Source: CAD feature listing. Evaluate the final solid. Frame: model axes, mm. Face numbers are marked on the shaded views. A direction names the side the tool comes from. Round coordinates to 2 decimals unless told otherwise and drop trailing zeros. Order: outer loops, then holes, each group sorted by start corner. A loop starts at its lowest first (then second) coordinate and runs counter-clockwise, first axis right, second up. Notation, with made-up numbers: (-2.75, 43) -> (40.25, 43) arc R10 ccw to (40.25, 49) -> close; hole circle Ø1 at (19, 37.5). An arc over 180 degrees is marked (long way). Answer as CSV lines item,"result". Start each with the question number.
(1) Set-up query: the marked faces 1 and 2. Return all of +Z, -Z, +X, -X, +Y, -Y with unobstructed straight access to the full face (end or side cutting, diameter ignored); none if empty.
(2) Section query D-D (z = 17.5). Output: boundary loops of the cut face in (x, y).
(3) Contact query for flat-ended pins moving along their axis: P1, Ø12, axis at y = -43.5, z = 64, coming from the -X side; P2, Ø4, axis at x = -90, y = -11, coming from the +Z side; P3, Ø10, axis at x = -128.5, y = -52.5, coming from the +Z side. Output: stop coordinate, or through.
(4) Section query A-A (x = -32). Output: boundary loops of the cut face in (y, z), plus the area to 3 significant figures.
(5) Pull-direction query (Z, two-part tool) for the marked faces 3, 4 and 5; classes: +Z half, -Z half, draft (parallel to the pull), parting line (faces both ways), or undercut.
(6) Section query C-C (y = -56.5). Output: boundary loops of the cut face in (x, z).
(7) Section query B-B (z = 63). Output: boundary loops of the cut face in (x, y).
(8) Line query: line 1 along X through (y, z) = (-7, 64); line 2 along X through (y, z) = (-75.5, 13); line 3 along Z through (x, y) = (-66.5, -90.5). Output: solid intervals per line, ascending. Write a range as from..to.
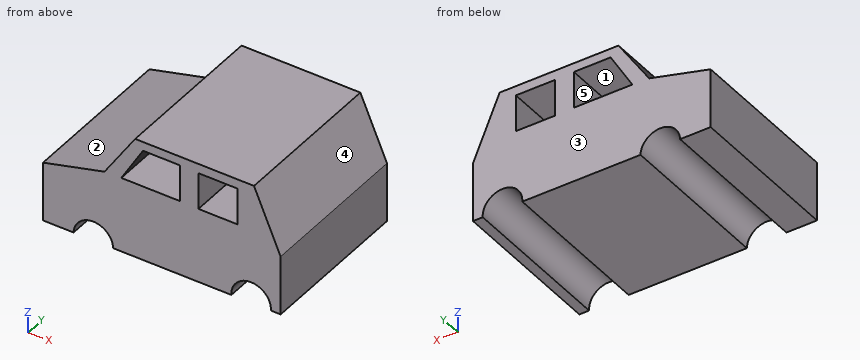
```python
from build123d import *

# Parameters (mm, degrees)
F1_DEPTH = 101.6
F3_DEPTH = 115.062
F4_W     = 25.222163
F4_H     = 23.562811
F5_DEPTH = 157.988
F6_R     = 12.7
F7_DEPTH = 195.834
F8_R     = 12.7
F9_DEPTH = 145.542


with BuildPart() as f1:
    # F0 (on Front) → F1 (new body)
    with BuildSketch(Plane.XZ):
        Polygon((-105.85011, 56.459235), (-145.276219, 46.419184), (-145.276219, 8.319184), (7.123781, 8.319184), (7.123781, 46.419184), (-9.965162, 86.073698), (-86.165162, 86.073698), align=None)
    extrude(amount=F1_DEPTH)

    # F2 (on Front) → F3 (cut)
    with BuildSketch(Plane.XZ):
        Polygon((-81.123598, 80.316171), (-95.062166, 56.75336), (-57.560787, 56.75336), (-57.560787, 80.316171), align=None)
    extrude(amount=F3_DEPTH, mode=Mode.SUBTRACT)

    # F4 (on Front) → F5 (cut)
    with BuildSketch(Plane.XZ):
        with Locations((-33.002364, 68.202894)):
            Rectangle(F4_W, F4_H)
    extrude(amount=F5_DEPTH, mode=Mode.SUBTRACT)

    # F6 (on Front) → F7 (cut)
    with BuildSketch(Plane.XZ):
        with Locations((-112.983182, 7.968382)):
            Circle(F6_R)
    extrude(amount=F7_DEPTH, mode=Mode.SUBTRACT)

    # F8 (on Front) → F9 (cut)
    with BuildSketch(Plane.XZ):
        with Locations((-11.795502, 9.144407)):
            Circle(F8_R)
    extrude(amount=F9_DEPTH, mode=Mode.SUBTRACT)


solid = f1.part
```
Answer block:
1,face 1,"+Y, -Y"
1,face 2,"+Z, -X, +Y, -Y"
2,outline,"(-145.28, -101.6) -> (-121.38, -101.6) -> (-121.38, 0) -> (-145.28, 0) -> close; (-104.59, -101.6) -> (-21.36, -101.6) -> (-21.36, 0) -> (-104.59, 0) -> close; (-2.23, -101.6) -> (7.12, -101.6) -> (7.12, 0) -> (-2.23, 0) -> close"
3,P1,"x = -104.83"
3,P2,"z = 83.31"
3,P3,"z = 51.96"
4,outline,"(-101.6, 8.32) -> (0, 8.32) -> (0, 56.42) -> (-101.6, 56.42) -> close; (-101.6, 79.98) -> (0, 79.98) -> (0, 86.07) -> (-101.6, 86.07) -> close"
4,area,"5,510 mm2"
5,face 3,"draft"
5,face 4,"+Z half"
5,face 5,"undercut"
6,outline,"(-145.28, 8.32) -> (-125.68, 8.32) arc R12.7 cw to (-100.29, 8.32) -> (-24.47, 8.32) arc R12.7 cw (long way) to (0.88, 8.32) -> (7.12, 8.32) -> (7.12, 46.42) -> (-9.97, 86.07) -> (-86.17, 86.07) -> (-105.85, 56.46) -> (-145.28, 46.42) -> close; hole (-95.06, 56.75) -> (-57.56, 56.75) -> (-57.56, 80.32) -> (-81.12, 80.32) -> close; hole (-45.61, 56.42) -> (-20.39, 56.42) -> (-20.39, 79.98) -> (-45.61, 79.98) -> close"
7,outline,"(-101.5, -101.6) -> (-91.37, -101.6) -> (-91.37, 0) -> (-101.5, 0) -> close; (-57.56, -101.6) -> (-45.61, -101.6) -> (-45.61, 0) -> (-57.56, 0) -> close; (-20.39, -101.6) -> (-0.02, -101.6) -> (-0.02, 0) -> (-20.39, 0) -> close"
8,line 1,"-100.84..-90.78, -57.56..-45.61, -20.39..-0.45"
8,line 2,"-145.28..-124.64, -101.32..-23.9, 0.31..7.12"
8,line 3,"8.32..56.75, 80.32..86.07"
